```python
from build123d import *

# Parameters (mm, degrees)
EXTRUDE_1_DEPTH = 1.5


with BuildPart() as part:
    # 草图1 → 凸台-拉伸1 (new body)
    with BuildSketch(Plane.XY):
        Polygon((2296.848886703, 1258.899784257), (2296.848886703, 1260.899784257), (2286.848886703, 1260.899784257), (2286.848886703, 1258.899784257), (2281.507070967, 1258.899784257), (2281.507070967, 1252.057968521), (2279.507070967, 1252.057968521), (2279.507070967, 1242.057968521), (2281.507070967, 1242.057968521), (2281.507070967, 1227.741599993), (2279.507070967, 1227.741599993), (2279.507070967, 1217.741599993), (2281.507070967, 1217.741599993), (2281.507070967, 1210.899784257), (2286.848886703, 1210.899784257), (2286.848886703, 1208.899784257), (2296.848886703, 1208.899784257), (2296.848886703, 1210.899784257), (2311.165255231, 1210.899784257), (2311.165255231, 1208.899784257), (2321.165255231, 1208.899784257), (2321.165255231, 1210.899784257), (2326.507070967, 1210.899784257), (2326.507070967, 1217.741599993), (2328.507070967, 1217.741599993), (2328.507070967, 1227.741599993), (2326.507070967, 1227.741599993), (2326.507070967, 1242.057968521), (2328.507070967, 1242.057968521), (2328.507070967, 1252.057968521), (2326.507070967, 1252.057968521), (2326.507070967, 1258.899784257), (2321.165255231, 1258.899784257), (2321.165255231, 1260.899784257), (2311.165255231, 1260.899784257), (2311.165255231, 1258.899784257), (2304.007070967, 1258.899784257), align=None)
        with BuildLine():
            ThreePointArc((2286.507070967, 1249.575559728), (2287.139332676, 1250.505489053), (2288.236608066, 1250.259500969))
            Line((2288.236608066, 1250.259500969), (2302.636365199, 1234.899764783))
            Line((2302.636365199, 1234.899764783), (2288.21378563, 1219.515654308))
            ThreePointArc((2288.21378563, 1219.515654308), (2287.124283961, 1219.299885135), (2286.507473515, 1220.223527434))
            Line((2286.507473515, 1220.223527434), (2286.507070967, 1249.575559728))
        make_face(mode=Mode.SUBTRACT)
        with BuildLine():
            Line((2290.723117316, 1219.267300568), (2304.007052849, 1233.437698409))
            Line((2304.007052849, 1233.437698409), (2317.335840115, 1219.220329728))
            ThreePointArc((2317.335840115, 1219.220329728), (2317.655344671, 1217.075780213), (2315.833356966, 1215.900392367))
            Line((2315.833356966, 1215.900392367), (2292.182284313, 1215.899458558))
            ThreePointArc((2292.182284313, 1215.899458558), (2290.347072244, 1217.104349752), (2290.723117316, 1219.267300568))
        make_face(mode=Mode.SUBTRACT)
        with BuildLine():
            ThreePointArc((2319.77790316, 1250.259120778), (2320.862789914, 1250.509889131), (2321.507070967, 1249.601722869))
            Line((2321.507070967, 1249.601722869), (2321.507070967, 1220.185997989))
            ThreePointArc((2321.507070967, 1220.185997989), (2320.857447426, 1219.287966637), (2319.778324446, 1219.540878969))
            Line((2319.778324446, 1219.540878969), (2305.377777603, 1234.89980238))
            Line((2305.377777603, 1234.89980238), (2319.77790316, 1250.259120778))
        make_face(mode=Mode.SUBTRACT)
        with BuildLine():
            Line((2304.007088097, 1236.36187164), (2290.722688538, 1250.531902224))
            ThreePointArc((2290.722688538, 1250.531902224), (2290.346584138, 1252.694842725), (2292.181763157, 1253.899784257))
            Line((2292.181763157, 1253.899784257), (2315.832835828, 1253.899499172))
            ThreePointArc((2315.832835828, 1253.899499172), (2317.659143856, 1252.714620558), (2317.32152184, 1250.563957934))
            Line((2317.32152184, 1250.563957934), (2304.007088097, 1236.36187164))
        make_face(mode=Mode.SUBTRACT)
    extrude(amount=EXTRUDE_1_DEPTH)


solid = part.part
```
Check sheet for the modelled part. Datum: model origin and axes. Units: mm. A direction names the side the tool comes from. Round coordinates to 2 decimals unless told otherwise and drop trailing zeros. Order: outer loops, then holes, each group sorted by start corner. A loop starts at its lowest first (then second) coordinate and runs counter-clockwise, first axis right, second up. Notation, with made-up numbers: (-20, 24.5) -> (15, 24.5) arc R17 cw to (15, 55.5) -> close; hole circle Ø6 at (69.25, -32). An arc over 180 degrees is marked (long way). One line per item, written item: value. Start each with the question number.
Q1. Cross-section at B-B (y = 1217). Record the boundary of the cut face in (x, z), and give its area (3 significant figures).
Q2. Gauge pin test, flat ends, axial feed: pin 1 Ø0.8 at (x, z) = (2305.5, 0.5) entering from -Y; pin 2 Ø0.8 at (y, z) = (1209.5, 0.5) entering from -X; pin 3 Ø0.8 at (y, z) = (1241, 1) entering from +X. Record the tip position at first contact, or that the pin passes through.
Q3. Cross-section at C-C (y = 1246.5). Record the boundary of the cut face in (x, z), and give its area (3 significant figures).
Q4. Set-up check for faces 1 (the face through (2290.36, 1217.075, 0.74)), 2 (the face through (2321.165, 1260, 1)), 3 (the face through (2326.507, 1235, 1)), 4 (the face through (2280, 1217.742, 1)): record each of +Z, -Z, +X, -X, +Y, -Y from which the full face is reachable in a straight line by a thin tool's end or side.
Q5. Cross-section at D-D (x = 2306.5). Record the boundary of the cut face in (y, z).
Q6. Thickness scan on line 1 (X direction, y = 1232, z = 0.4); line 2 (X direction, y = 1229.5, z = 1.05); line 3 (Y direction, x = 2297, z = 0.8). Record the ranges inside material, lowest first.
Q7. Mould release check, pull along Y, two halves, no side actions. Record for faces 5 (the face through (2317.646, 1252.744, 0.74)), 6 (the face through (2328.507, 1223, 1)), 7 (the face through (2292, 1208.9, 1)): pulls with the +Y half, pulls with the -Y half, needs draft (parallel to the pull), parting line crosses it, or undercut.
Q8. Cross-section at A-A (x = 2289). Record the boundary of the cut face in (y, z).
Completed:
1. outline: (2281.51, 0) -> (2290.4, 0) -> (2290.4, 1.5) -> (2281.51, 1.5) -> close; (2317.62, 0) -> (2326.51, 0) -> (2326.51, 1.5) -> (2317.62, 1.5) -> close
1. area: 26.7 mm²
2. pin 1: stops at y = 1210.9
2. pin 2: stops at x = 2286.85
2. pin 3: stops at x = 2326.51
3. outline: (2279.51, 0) -> (2286.51, 0) -> (2286.51, 1.5) -> (2279.51, 1.5) -> close; (2291.76, 0) -> (2294.5, 0) -> (2294.5, 1.5) -> (2291.76, 1.5) -> close; (2313.51, 0) -> (2316.25, 0) -> (2316.25, 1.5) -> (2313.51, 1.5) -> close; (2321.51, 0) -> (2328.51, 0) -> (2328.51, 1.5) -> (2321.51, 1.5) -> close
3. area: 29.2 mm²
4. face 1: +Z, -Z
4. face 2: +Z, -Z, +X, +Y
4. face 3: +Z, -Z, +X
4. face 4: +Z, -Z, -X, -Y
5. outline: (1210.9, 0) -> (1215.9, 0) -> (1215.9, 1.5) -> (1210.9, 1.5) -> close; (1230.78, 0) -> (1233.7, 0) -> (1233.7, 1.5) -> (1230.78, 1.5) -> close; (1236.1, 0) -> (1239.02, 0) -> (1239.02, 1.5) -> (1236.1, 1.5) -> close; (1253.9, 0) -> (1258.9, 0) -> (1258.9, 1.5) -> (1253.9, 1.5) -> close
6. line 1: x = 2281.51 to 2286.51, 2299.92 to 2302.66, 2305.35 to 2308.1, 2321.51 to 2326.51
6. line 2: x = 2281.51 to 2286.51, 2297.57 to 2300.32, 2307.7 to 2310.44, 2321.51 to 2326.51
6. line 3: y = 1210.9 to 1215.9, 1225.96 to 1228.89, 1240.91 to 1243.84, 1253.9 to 1258.9
7. face 5: undercut
7. face 6: needs draft
7. face 7: pulls with the -Y half
8. outline: (1208.9, 0) -> (1220.35, 0) -> (1220.35, 1.5) -> (1208.9, 1.5) -> close; (1249.45, 0) -> (1260.9, 0) -> (1260.9, 1.5) -> (1249.45, 1.5) -> close
